from build123d import *

# Parameters (mm, degrees)
EXTRUDE_1_DEPTH     = 200
SKETCH_2_3_W        = 16
SKETCH_2_3_H        = 650
EXTRUDE_2_DEPTH     = 140
SKETCH_2_4_W        = 200
SKETCH_2_4_H        = 313
EXTRUDE_3_DEPTH     = 6
EXTRUDE_4_DEPTH     = 100
SKETCH_3_R          = 15.5
CUT_EXTRUDE_5_DEPTH = 1353.439647452
SKETCH_6_R          = 15.5
CUT_EXTRUDE_6_DEPTH = 1353.439647452
SKETCH_7_R          = 15.5
CUT_EXTRUDE_7_DEPTH = 16
SKETCH_8_R          = 15.5
CUT_EXTRUDE_8_DEPTH = 12


with BuildPart() as part:
    # 草图2 → 拉伸1 (new, symmetric)
    with BuildSketch(Plane.XY):
        Polygon((0, 0), (0, 12), (-1228, 12), (-1228, 0), (-1028, 0), align=None)
    extrude(amount=EXTRUDE_1_DEPTH, both=True)

    # 草图2<3> → 拉伸2 (add, symmetric)
    with BuildSketch(Plane.XY):
        with Locations((-1236, 12)):
            Rectangle(SKETCH_2_3_W, SKETCH_2_3_H)
    extrude(amount=EXTRUDE_2_DEPTH, both=True)

    # 草图2<4> → 拉伸3 (add, symmetric)
    with BuildSketch(Plane.XY):
        Polygon((0, 473), (-1080, 473), (-1149.781745931, 403.218254069), (-1228, 325), (-1228, 12), (0, 12), align=None)
        with Locations((-1128, -156.5)):
            Rectangle(SKETCH_2_4_W, SKETCH_2_4_H)
    extrude(amount=EXTRUDE_3_DEPTH, both=True)

    # 草图2<5> → 拉伸4 (add, symmetric)
    with BuildSketch(Plane.XY):
        Polygon((-1149.781745931, 403.218254069), (-1080, 473), (-1096, 473), (-1157.781745931, 411.218254069), align=None)
        Polygon((-1096, 473), (-1080, 473), (0, 473), (0, 489), (-1080, 489), align=None)
    extrude(amount=EXTRUDE_4_DEPTH, both=True)

    # 草图3 → 拉伸5 (cut, through all)
    with BuildSketch(Plane.XY.offset(6)):
        with Locations((-990, 387)):
            Circle(SKETCH_3_R)
        with Locations((-810, 387)):
            Circle(SKETCH_3_R)
        with Locations((-990, 287)):
            Circle(SKETCH_3_R)
        with Locations((-810, 287)):
            Circle(SKETCH_3_R)
        with Locations((-990, 187)):
            Circle(SKETCH_3_R)
        with Locations((-810, 187)):
            Circle(SKETCH_3_R)
    extrude(amount=-CUT_EXTRUDE_5_DEPTH, mode=Mode.SUBTRACT)

    # 草图6 → 拉伸6 (cut, through all)
    with BuildSketch(Plane.XY.offset(6)):
        with Locations((-1122.413652083, -100.738221798)):
            Circle(SKETCH_6_R)
        with Locations((-1052.267682131, -157.125657451)):
            Circle(SKETCH_6_R)
        with Locations((-1122.413652083, -205.738221798)):
            Circle(SKETCH_6_R)
        with Locations((-1052.267682131, -262.125657451)):
            Circle(SKETCH_6_R)
    extrude(amount=-CUT_EXTRUDE_6_DEPTH, mode=Mode.SUBTRACT)

    # 草图7 → 拉伸7 (cut)
    with BuildSketch(Plane.ZY.offset(1244)):
        Polygon((-110, 12), (-110, 337), (-140, 337), (-140, -18), align=None)
        Polygon((140, 337), (110, 337), (110, 12), (140, -18), align=None)
        with Locations((60, 257)):
            Circle(SKETCH_7_R)
        with Locations((-60, 257)):
            Circle(SKETCH_7_R)
        with Locations((60, 67)):
            Circle(SKETCH_7_R)
        with Locations((-60, 67)):
            Circle(SKETCH_7_R)
        with Locations((95, -268)):
            Circle(SKETCH_7_R)
        with Locations((-95, -268)):
            Circle(SKETCH_7_R)
        with Locations((95, -168)):
            Circle(SKETCH_7_R)
        with Locations((-95, -168)):
            Circle(SKETCH_7_R)
        with Locations((95, -68)):
            Circle(SKETCH_7_R)
        with Locations((-95, -68)):
            Circle(SKETCH_7_R)
    extrude(amount=-CUT_EXTRUDE_7_DEPTH, mode=Mode.SUBTRACT)

    # 草图8 → 拉伸8 (cut)
    with BuildSketch(Plane.XZ):
        Polygon((-1228, 110), (-1138, 200), (-1228, 200), align=None)
        Polygon((-1228, -200), (-1138, -200), (-1228, -110), align=None)
        with Locations(Location((-1122.413652083, -97.738221798, 0), (0, 0, 270))):
            Circle(SKETCH_8_R)
        with Locations(Location((-1052.267682131, -154.125657451, 0), (0, 0, 270))):
            Circle(SKETCH_8_R)
        with Locations(Location((-1052.267682131, 154.125657451, 0), (0, 0, 90))):
            Circle(SKETCH_8_R)
        with Locations(Location((-1122.413652083, 97.738221798, 0), (0, 0, 90))):
            Circle(SKETCH_8_R)
        with Locations(Location((-191.732317869, -154.125657451, 0), (0, 0, 90))):
            Circle(SKETCH_8_R)
        with Locations(Location((-121.586347917, -97.738221798, 0), (0, 0, 90))):
            Circle(SKETCH_8_R)
        with Locations(Location((-191.732317869, 154.125657451, 0), (0, 0, 270))):
            Circle(SKETCH_8_R)
        with Locations(Location((-121.586347917, 97.738221798, 0), (0, 0, 270))):
            Circle(SKETCH_8_R)
    extrude(amount=-CUT_EXTRUDE_8_DEPTH, mode=Mode.SUBTRACT)

    # 镜向1: part across plane


with BuildPart() as part_1:
    add(part.part)
    add(part.part.mirror(Plane(origin=(0, 0, 200), x_dir=(0, 0, 1), z_dir=(1, 0, 0))))


solid = part_1.part
Check sheet for the modelled part. Datum: model origin and axes. Units: mm. A direction names the side the tool comes from. Give positions to 0.01 mm unless a question says otherwise; leave off trailing zeros. Order: outer loops, then holes, each group sorted by start corner. A loop starts at its lowest first (then second) coordinate and runs counter-clockwise, first axis right, second up. Notation, with made-up numbers: M 62.5,16 L 111.5,16 A13 cw 111.5,29 Z; hole C -3.75,81.25 d3. An arc over 180 degrees is marked long. Answer as CSV lines item,"result". Start each with the question number.
Item 1: Cross-section at B-B on x = -464.5. Enter the section's corners in (y, z).
Item 2: Thickness scan on line 1 (Y direction, x = 810, z = 1); line 2 (Y direction, x = 692, z = 45.5); line 3 (X direction, y = -30.5, z = 132.5). Record the ranges inside material, lowest first. Write a range as [from, to].
Item 3: Tool access check on faces 4 (the face through (1115, 438, -52)), 5 (the face through (-1115, 438, 54)), 6 (the face through (1129, -154, -6)), 7 (the face through (5, 478, 100)), 8 (the face through (1228, -153, 74)). Record the directions out of +Z, -Z, +X, -X, +Y, -Y that give a thin tool (end or side, any length) a straight path to the whole face; none if there is none.
Item 4: Mould release check, pull along Y, two halves, no side actions. Record for faces 1 (the face through (-1129, -154, -6)), 2 (the face through (-1118, 451, 1)), 3 (the face through (1115, 438, 54)): +Y half, -Y half, draft (parallel to the pull), parting line (faces both ways), or undercut.
Item 5: Gauge pin test, flat ends, axial feed: P1, Ø8, axis at x = 103.5, y = 317.5, coming from the -Z side; P2, Ø17.5, axis at x = -1236, y = -196.5, coming from the -Z side; P3, Ø17.5, axis at x = 1240, z = -55, coming from the +Y side. Record the tip position at first contact, or that the pin passes through.
Item 6: Cross-section at A-A on y = 141.5. Enter the section's corners in (x, z), plus the area to 3 significant figures.
Established:
1,outline,"M 0,-200 L 12,-200 L 12,-6 L 473,-6 L 473,-100 L 489,-100 L 489,100 L 473,100 L 473,6 L 12,6 L 12,200 L 0,200 Z"
2,line 1,"y = [0, 171.5], [202.5, 271.5], [302.5, 371.5], [402.5, 489]"
2,line 2,"y = [0, 12], [473, 489]"
2,line 3,"x = [-1244, -1228], [1228, 1244]"
3,face 4,"-Z"
3,face 5,"+Z"
3,face 6,"-Z, -Y"
3,face 7,"+Z, +X, -X, +Y"
3,face 8,"+Z, -Y"
4,face 1,"draft"
4,face 2,"+Y half"
4,face 3,"undercut"
5,P1,"stops at z = -6"
5,P2,"stops at z = -140"
5,P3,"stops at y = 337"
6,outline,"M -1244,-110 L -1228,-110 L -1228,-6 L 1228,-6 L 1228,-110 L 1244,-110 L 1244,110 L 1228,110 L 1228,6 L -1228,6 L -1228,110 L -1244,110 Z"
6,area,"36,500 mm^2"
